Autodesk Inventor part; units mm, degrees
ref_plane "YZ Plane" through (0, 0, 0) normal (1, 0, 0) x (0, 1, 0)
ref_plane "XZ Plane" through (0, 0, 0) normal (0, 1, 0) x (-1, 0, 0)
ref_plane "XY Plane" through (0, 0, 0) normal (0, 0, 1) x (1, 0, 0)
sketch "Sketch1" plane through (0, 0, 0) normal (0, 0, 1) x (1, 0, 0)
  circle A0 centre (4.056, -0.4) radius 1.05
  line L0 (-10.5, -3.4) -> (-10.5, 3.4)
  line L1 (4.056, -3.4) -> (-10.5, -3.4)
  arc A1 (4.056, -3.4) -> (7.056, -0.4) centre (4.056, -0.4) ccw
  line L2 (9.056, -0.4) -> (7.056, -0.4)
  line L3 (10.5, 1.4) -> (9.056, -0.4)
  line L4 (10.5, 3.4) -> (10.5, 1.4)
  line L5 (-10.5, 3.4) -> (10.5, 3.4)
  point P0 (0, 0)
sketch "Sketch2" plane through (0, 0, 0) normal (0, 0, 1) x (1, 0, 0)
  arc A0 (-11.5298, 4.6) -> (-12.3624, -1.6977) centre (2.056, -0.4) ccw
  line L0 (4.056, -0.4) -> (2.056, -0.4) construction
  circle A1 centre (-10.944, 6.6) radius 2 construction
  line L1 (-11.5298, 4.6) -> (-8.944, 4.6)
  line L2 (-11.5298, 4.6) -> (4.056, -0.4) construction
  line L3 (4.056, -0.4) -> (-12.3624, -1.6977) construction
  circle A2 centre (-12.944, 6.0142) radius 2 construction
  line L4 (-12.944, 6.0142) -> (-11.5298, 4.6) construction
  line L5 (-12.944, 6.0142) -> (-10.944, 6.0142) construction
  line L6 (4.056, -3.4) -> (-10.5, -3.4) construction
  arc A3 (-12.3624, -1.6977) -> (-10.5, -3.4) centre (-10.5, -1.5301) ccw
  point P0 (0, 0)
  point P1 (-8.944, 6.6)
  dimension "d1" = 4
  dimension "d0" = 2
  dimension "d2" = 7
  dimension "d3" = 15
  dimension "d11" = 45
  dimension "d12" = 2
sketch "Sketch3" plane through (0, 0, 0) normal (0, 0, 1) x (1, 0, 0)
  arc A0 (-11.5298, 4.6) -> (-12.3624, -1.6977) centre (2.056, -0.4) ccw
  line L0 (-11.5298, 4.6) -> (-8.944, 4.6)
  line L1 (10.5, 5) -> (10.5, 1.4)
  line L2 (10.5, 3.4) -> (10.5, 1.4) construction
  circle A1 centre (4.056, -0.4) radius 1.05
  line L3 (4.056, -3.4) -> (-10.5, -3.4)
  arc A2 (4.056, -3.4) -> (7.056, -0.4) centre (4.056, -0.4) ccw
  line L4 (9.056, -0.4) -> (7.056, -0.4)
  line L5 (10.5, 1.4) -> (9.056, -0.4)
  arc A3 (-12.3624, -1.6977) -> (-10.5, -3.4) centre (-10.5, -1.5301) ccw
  line L6 (-8.944, 4.6) -> (-6.944, 4.6)
  line L7 (-6.944, 4.6) -> (-6.944, 5)
  line L8 (-6.944, 5) -> (10.5, 5)
  line L9 (-10.5, 3.4) -> (10.5, 3.4) construction
  point P0 (0, 0)
  dimension "d18" = 1.6
  dimension "d19" = 2
extrude "Extrusion1" add sketch "Sketch3" along normal blind 2
sketch "Sketch4" plane through (0, 0, 0) normal (0, 0, -1) x (-1, 0, 0)
  arc A0 (12.3624, -1.6977) -> (11.5298, 4.6) centre (-2.056, -0.4) ccw
  line L0 (6.944, 4.6) -> (11.5298, 4.6)
  line L1 (-10.5, 1.4) -> (-10.5, 5)
  line L2 (-9.056, -0.4) -> (-10.5, 1.4)
  line L3 (-7.056, -0.4) -> (-9.056, -0.4)
  arc A1 (-7.056, -0.4) -> (-4.056, -3.4) centre (-4.056, -0.4) ccw
  line L4 (10.5, -3.4) -> (-4.056, -3.4)
  arc A2 (10.5, -3.4) -> (12.3624, -1.6977) centre (10.5, -1.5301) ccw
  circle A3 centre (-4.056, -0.4) radius 1.05
  line L5 (6.944, 5) -> (6.944, 4.6)
  line L6 (-10.5, 5) -> (6.944, 5)
  line L7 (-10.5, 5) -> (6.944, 5)
  line L8 (-10.5, 1.4) -> (-10.5, 5)
  line L9 (6.944, 5) -> (-10.5, 5)
  line L10 (-10.5, 5) -> (-10.5, 3.4)
  line L11 (-10.5, 3.4) -> (6.944, 3.4)
  line L12 (6.944, 3.4) -> (6.944, 5)
  line L13 (-10.5, 1.4) -> (-10.5, 5)
extrude "Extrusion2" add sketch "Sketch4" along normal blind 2 contours L12 L11 L1 L6 L5
sketch "Sketch5" plane through (0, 0, 0) normal (0, 0, 1) x (1, 0, 0)
  circle A0 centre (-10.944, 6.6) radius 2 construction
  point P0 (0, 0)
properties part number "Capping_RotationGuide"
Read the model definition and answer for the solid it produces. Units are mm, in the model's axes. A direction names the side the tool comes from. Round coordinates to 2 decimals unless told otherwise and drop trailing zeros. Order: outer loops, then holes, each group sorted by start corner. A loop starts at its lowest first (then second) coordinate and runs counter-clockwise, first axis right, second up.
1) The part is cut by section B-B on x = -9.5. Write down the section's boundary in (y, z), plus the area to 3 significant figures.
2) Flat-ended cylindrical pins translate along their axes: pin 1 (0.5 mm diameter, centred on y = 4, z = -0.5, fed in from -X); pin 2 (0.6 mm diameter, centred on x = -10, z = 1, fed in from +Y); pin 3 (0.6 mm diameter, centred on x = 6, z = -1.5, fed in from -Y). Find the tip coordinate at first contact, or state that the pin passes through.
3) The mould has two halves that part along Y. Classify faces 1 (the face through (2, 5, 0)), 2 (the face through (5.058, -0.715, 0.986)), 3 (the face through (6.2, -2.5, 1)): released by +Y, released by -Y, zero draft, split by the parting line, or undercut.
4) The part is cut by section C-C on y = 2. Write down the section's boundary in (x, z).
5) The part is cut by section A-A on z = 1.35. Write down the section's boundary in (x, y).
6) The part is cut by section D-D on x = -5.25. Write down the section's boundary in (y, z).
7) Straight lines are drawn through the part: L1, parallel to Z at x = 7.5, y = 3.25; L2, parallel to Y at x = 8.5, z = 1; L3, parallel to Y at x = -6, z = -0.7. For each, find the intervals that lie inside material, in ascending order.
8) For faces 4 (the face through (10.5, 4, 0)), 5 (the face through (8, -0.4, 1)), 6 (the face through (2, 3.4, -1)), 7 (the face through (-9, 4.6, 1)), determine the directions among +Z, -Z, +X, -X, +Y, -Y from which every point of the face is accessible in a straight line to the end or side of a thin tool.
Resolved:
1. outline: (-3.4, 0) - (4.6, 0) - (4.6, 2) - (-3.4, 2) - close
1. area: 16.0 mm2
2. pin 1: stops at x = -6.94
2. pin 2: stops at y = 4.6
2. pin 3: stops at y = 3.4
3. face 1: released by +Y
3. face 2: undercut
3. face 3: released by -Y
4. outline: (-12.22, 0) - (10.5, 0) - (10.5, 2) - (-12.22, 2) - close
5. outline: (-12.36, -1.7) arc R1.87 ccw to (-10.5, -3.4) - (4.06, -3.4) arc R3 ccw to (7.06, -0.4) - (9.06, -0.4) - (10.5, 1.4) - (10.5, 5) - (-6.94, 5) - (-6.94, 4.6) - (-11.53, 4.6) arc R14.48 ccw to start; hole circle Ø2.1 at (4.06, -0.4)
6. outline: (-3.4, 0) - (3.4, 0) - (3.4, -2) - (5, -2) - (5, 2) - (-3.4, 2) - close
7. L1: z = 0 to 2
7. L2: y = -0.4 to 5
7. L3: y = 3.4 to 5
8. face 4: +Z, -Z, +X, +Y, -Y
8. face 5: +Z, -Z, +X, -Y
8. face 6: -Z, +X, -X, -Y
8. face 7: +Z, -Z, -X, +Y
